```python
from build123d import *

# Parameters (mm, degrees)
SKETCH1_R           = 16
SKETCH1_R_2         = 7.1
SKETCH1_R_3         = 2
SKETCH1_R_4         = 2.1
BOSS_EXTRUDE1_DEPTH = 8
SKETCH2_R           = 7.55
CUT_EXTRUDE1_DEPTH  = 1.08


with BuildPart() as part:
    # Sketch1 → Boss-Extrude1 (new body)
    with BuildSketch(Plane(origin=(0, 0, 0), x_dir=(1, 0, 0), z_dir=(0, 1, 0))):
        Circle(SKETCH1_R)
        Circle(SKETCH1_R_2, mode=Mode.SUBTRACT)
        with Locations((0, 11.313708499)):
            Circle(SKETCH1_R_3, mode=Mode.SUBTRACT)
        with Locations((-11.313708499, 0)):
            Circle(SKETCH1_R_3, mode=Mode.SUBTRACT)
        with Locations((0, -11.313708499)):
            Circle(SKETCH1_R_3, mode=Mode.SUBTRACT)
        with Locations((11.313708499, 0)):
            Circle(SKETCH1_R_3, mode=Mode.SUBTRACT)
        with Locations((-8, -8)):
            Circle(SKETCH1_R_4, mode=Mode.SUBTRACT)
        with Locations((8, -8)):
            Circle(SKETCH1_R_4, mode=Mode.SUBTRACT)
        with Locations((8, 8)):
            Circle(SKETCH1_R_4, mode=Mode.SUBTRACT)
        with Locations((-8, 8)):
            Circle(SKETCH1_R_4, mode=Mode.SUBTRACT)
    extrude(amount=BOSS_EXTRUDE1_DEPTH)

    # Sketch2 → Cut-Extrude1 (cut)
    with BuildSketch(Plane(origin=(0, 8, 0), x_dir=(1, 0, 0), z_dir=(0, 1, 0))):
        Circle(SKETCH2_R)
    extrude(amount=-CUT_EXTRUDE1_DEPTH, mode=Mode.SUBTRACT)


solid = part.part
```
Verification items for the finished model (mm, model axes). A direction names the side the tool comes from. Coordinates: 2 decimals unless noted, no trailing zeros. Loops run counter-clockwise (first coordinate to the right, second up) from the corner with the lowest first, then second, coordinate; pieces in that order, holes last. Notation, with made-up numbers: (28.25, -26.5) -> (50.25, -26.5) arc R18 ccw to (50.25, -15.5) -> close; hole circle Ø1 at (40, 7.5). An arc over 180 degrees is marked (long way). Answer in a Markdown table with one row per item. Add a question column.
1. Material ranges on probe 1 along Z at (x, y) = (0, 2.5); probe 2 along Z at (x, y) = (-8, 4.5), recorded low to high. Write a range as [from, to].
2. Draft check along X on faces 3 (the face through (7, 8, -4)), 4 (the face through (-3.47, 3.94, 15.62)), 5 (the face through (7.727, 3.944, -10.082)). Enter one of: +X half, -X half, draft (parallel to the pull), parting line (faces both ways), or undercut.
3. Access from +Z, -Z, +X, -X, +Y, -Y to the whole of each face (thin tool, end or side, straight path). Record for faces 1 (the face through (-1.64, 7.47, 7.37)), 2 (the face through (7.727, 3.944, 5.918)).
4. Section check B-B, the plane x = 5.5. Enter the section's corners in (y, z).
5. Depth check by flat-ended pin: P1, Ø2.5, axis at x = 0, z = -11.31, coming from the +Y side; P2, Ø1, axis at y = 6, z = 3.5, coming from the -X side; P3, Ø4, axis at x = 4.5, y = 7, coming from the -Z side; P4, Ø1.5, axis at x = 11.5, y = 4.5, coming from the +Z side. Enter the tip coordinate at first touch or a pass-through.
6. Section check C-C, the plane z = -8.5. Enter the section's corners in (x, y).
7. Section check A-A, the plane z = 0. Enter the section's corners in (x, y), then the cut area to 3 significant figures.
8. Section check D-D, the plane y = 4.5. Give the number of separate pieces and of enclosed holes in the cut face, then the cut area to 3 significant figures.
Derived:
| question | item | result |
|---|---|---|
| 1 | probe 1 | z = [-16, -13.31], [-9.31, -7.1], [7.1, 9.31], [13.31, 16] |
| 1 | probe 2 | z = [-13.86, -10.1], [-5.9, 5.9], [10.1, 13.86] |
| 2 | face 3 | draft |
| 2 | face 4 | parting line |
| 2 | face 5 | undercut |
| 3 | face 1 | +Y |
| 3 | face 2 | +Y, -Y |
| 4 | outline | (0, -15.02) -> (8, -15.02) -> (8, -5.17) -> (6.92, -5.17) -> (6.92, -4.49) -> (0, -4.49) -> close; (0, 4.49) -> (6.92, 4.49) -> (6.92, 5.17) -> (8, 5.17) -> (8, 15.02) -> (0, 15.02) -> close |
| 5 | P1 | passes through |
| 5 | P2 | stops at x = -15.72 |
| 5 | P3 | stops at z = -15.8 |
| 5 | P4 | stops at z = 11.85 |
| 6 | outline | (-13.56, 0) -> (-10.04, 0) -> (-10.04, 8) -> (-13.56, 8) -> close; (-5.96, 0) -> (5.96, 0) -> (5.96, 8) -> (-5.96, 8) -> close; (10.04, 0) -> (13.56, 0) -> (13.56, 8) -> (10.04, 8) -> close |
| 7 | outline | (-16, 0) -> (-13.31, 0) -> (-13.31, 8) -> (-16, 8) -> close; (-9.31, 0) -> (-7.1, 0) -> (-7.1, 6.92) -> (-7.55, 6.92) -> (-7.55, 8) -> (-9.31, 8) -> close; (7.1, 0) -> (9.31, 0) -> (9.31, 8) -> (7.55, 8) -> (7.55, 6.92) -> (7.1, 6.92) -> close; (13.31, 0) -> (16, 0) -> (16, 8) -> (13.31, 8) -> close |
| 7 | area | 77.4 mm² |
| 8 | separate pieces | 1 |
| 8 | enclosed holes | 9 |
| 8 | area | 540 mm² |
